Check sheet for the modelled part. Datum: model origin and axes. Units: mm. Face numbers are marked on the shaded views. Round coordinates to 2 decimals unless told otherwise and drop trailing zeros. Write each loop counter-clockwise with the first axis right and the second up, starting at its lowest first coordinate (ties: lowest second). Pieces come first, ordered by that corner, then holes. Notation, with made-up numbers: (16.25, 6) -> (44.25, 6) arc R20 ccw to (44.25, 44) -> close; hole circle Ø10 at (8, 52). An arc over 180 degrees is marked (long way). One line per item, written item: value.
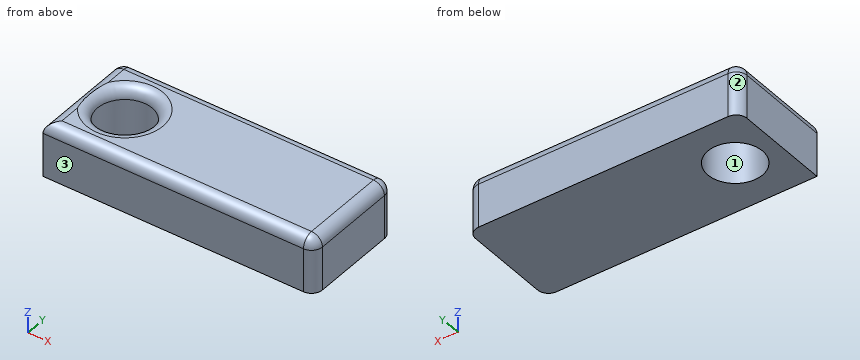
from build123d import *

# Parameters (mm, degrees)
F0_W         = 124.3421025574
F0_H         = 48.8486886024
F1_DEPTH     = 25
F3_D         = 25
F4_T1_DEPTH  = 149.3421025574
F4_T3_DEPTH  = 73.8486886024
F5_T1_DEPTH  = 32.5
F5_S5_W      = 5
F5_S5_H      = 5
F5_T6_DEPTH  = 5
F6_T1_DEPTH  = 32.5
F6_S5_W      = 5
F6_S5_H      = 5
F6_T6_DEPTH  = 5
F6_S11_W     = 5
F6_S11_H     = 5
F6_T12_DEPTH = 5


# Not quite as in the source:
# - a fillet or chamfer that OpenCascade refuses, or shapes differently, is made with other operations: its cross-section is extruded or revolved along the edge and cut away or added


with BuildPart() as f1:
    # F0 (on Top) → F1 (new body)
    with BuildSketch(Plane.XY):
        with Locations((-25.8323382586, 0)):
            Rectangle(F0_W, F0_H)
    extrude(amount=F1_DEPTH)

    # F3 (through all)
    with Locations(Plane.XY.offset(25)):
        with Locations((-68.3952495456, 0)):
            Hole(F3_D / 2)

    # F4: fillet of radius 5 on 5 edges, made by hand

    # F4_s2 → F4_t1 (cut)
    with BuildSketch(Plane.YZ.offset(-100.5033895373)):
        with BuildLine():
            ThreePointArc((24.4243443012, 20), (22.9598782072, 23.5355339059), (19.4243443012, 25))
            Line((19.4243443012, 25), (24.4243443012, 25))
            Line((24.4243443012, 25), (24.4243443012, 20))
        make_face()
        with BuildLine():
            ThreePointArc((-19.4243443012, 25), (-22.9598782072, 23.5355339059), (-24.4243443012, 20))
            Line((-24.4243443012, 20), (-24.4243443012, 25))
            Line((-24.4243443012, 25), (-19.4243443012, 25))
        make_face()
    extrude(amount=F4_T1_DEPTH, mode=Mode.SUBTRACT)

    # F4_s4 → F4_t3 (cut)
    with BuildSketch(Plane.XZ.offset(-36.9243443012)):
        with BuildLine():
            ThreePointArc((36.3387130201, 20), (34.874246926, 23.5355339059), (31.3387130201, 25))
            Line((31.3387130201, 25), (36.3387130201, 25))
            Line((36.3387130201, 25), (36.3387130201, 20))
        make_face()
        with BuildLine():
            ThreePointArc((-88.0033895373, 20), (-86.5389234433, 23.5355339059), (-83.0033895373, 25))
            Line((-83.0033895373, 25), (-88.0033895373, 25))
            Line((-88.0033895373, 25), (-88.0033895373, 20))
        make_face()
    extrude(amount=F4_T3_DEPTH, mode=Mode.SUBTRACT)

    # F4_s5 → F4_t6 (revolve, cut)
    with BuildSketch(Plane.XZ):
        with BuildLine():
            ThreePointArc((-50.8952495456, 25), (-54.4307834515, 23.5355339059), (-55.8952495456, 20))
            Line((-55.8952495456, 20), (-55.8952495456, 25))
            Line((-55.8952495456, 25), (-50.8952495456, 25))
        make_face()
    revolve(axis=Axis((-68.3952495456, 0, 25), (0, 0, 1)), mode=Mode.SUBTRACT)

    # F5: fillet of radius 5 on 1 edges, made by hand

    # F5_s2 → F5_t1 (cut)
    with BuildSketch(Plane.XY.offset(-12.5)):
        with BuildLine():
            ThreePointArc((36.3387130201, -19.4243443012), (34.874246926, -22.9598782072), (31.3387130201, -24.4243443012))
            Line((31.3387130201, -24.4243443012), (36.3387130201, -24.4243443012))
            Line((36.3387130201, -24.4243443012), (36.3387130201, -19.4243443012))
        make_face()
    extrude(amount=F5_T1_DEPTH, mode=Mode.SUBTRACT)


with BuildPart() as f5_tool4:
    # F5_s5 → F5_t6 (new body)
    with BuildSketch(Plane.YZ.offset(31.3387130201)):
        with Locations((-21.9243443012, 22.5)):
            Rectangle(F5_S5_W, F5_S5_H)
    extrude(amount=F5_T6_DEPTH)

    # F5_s7 → F5_t8 (revolve, cut)
    with BuildSketch(Plane(origin=(31.3387130201, -19.4243443012, 20), x_dir=(0, 0.7071067812, -0.7071067812), z_dir=(0, -0.7071067812, -0.7071067812))):
        with BuildLine():
            ThreePointArc((0, -5), (5, 0), (0, 5))
            Line((0, 5), (0, -5))
        make_face()
    revolve(axis=Axis((31.3387130201, -19.4243443012, 20), (1, 0, 0)), mode=Mode.SUBTRACT)


with BuildPart() as f1_1:
    add(f1.part)

    # F5_t3: cut F5_tool4
    add(f5_tool4.part, mode=Mode.SUBTRACT)

    # F6: fillet of radius 5 on 2 edges, made by hand

    # F6_s2 → F6_t1 (cut)
    with BuildSketch(Plane.XY.offset(-12.5)):
        with BuildLine():
            ThreePointArc((-83.0033895373, 24.4243443012), (-86.5389234433, 22.9598782072), (-88.0033895373, 19.4243443012))
            Line((-88.0033895373, 19.4243443012), (-88.0033895373, 24.4243443012))
            Line((-88.0033895373, 24.4243443012), (-83.0033895373, 24.4243443012))
        make_face()
        with BuildLine():
            ThreePointArc((31.3387130201, 24.4243443012), (34.874246926, 22.9598782072), (36.3387130201, 19.4243443012))
            Line((36.3387130201, 19.4243443012), (36.3387130201, 24.4243443012))
            Line((36.3387130201, 24.4243443012), (31.3387130201, 24.4243443012))
        make_face()
    extrude(amount=F6_T1_DEPTH, mode=Mode.SUBTRACT)


with BuildPart() as f6_tool4:
    # F6_s5 → F6_t6 (new body)
    with BuildSketch(Plane.XZ.offset(-19.4243443012)):
        with Locations((33.8387130201, 22.5)):
            Rectangle(F6_S5_W, F6_S5_H)
    extrude(amount=-F6_T6_DEPTH)

    # F6_s7 → F6_t8 (revolve, cut)
    with BuildSketch(Plane(origin=(31.3387130201, 19.4243443012, 20), x_dir=(-0.7071067812, 0, -0.7071067812), z_dir=(0.7071067812, 0, -0.7071067812))):
        with BuildLine():
            ThreePointArc((0, -5), (5, 0), (0, 5))
            Line((0, 5), (0, -5))
        make_face()
    revolve(axis=Axis((31.3387130201, 19.4243443012, 20), (0, 1, 0)), mode=Mode.SUBTRACT)


with BuildPart() as f1_2:
    add(f1_1.part)

    # F6_t3: cut F6_tool4
    add(f6_tool4.part, mode=Mode.SUBTRACT)


with BuildPart() as f6_tool10:
    # F6_s11 → F6_t12 (new body)
    with BuildSketch(Plane.XZ.offset(-19.4243443012)):
        with Locations((-85.5033895373, 22.5)):
            Rectangle(F6_S11_W, F6_S11_H)
    extrude(amount=-F6_T12_DEPTH)

    # F6_s13 → F6_t14 (revolve, cut)
    with BuildSketch(Plane(origin=(-83.0033895373, 19.4243443012, 20), x_dir=(0.7071067812, 0, -0.7071067812), z_dir=(0.7071067812, 0, 0.7071067812))):
        with BuildLine():
            ThreePointArc((0, -5), (5, 0), (0, 5))
            Line((0, 5), (0, -5))
        make_face()
    revolve(axis=Axis((-83.0033895373, 19.4243443012, 20), (0, 1, 0)), mode=Mode.SUBTRACT)


with BuildPart() as f1_3:
    add(f1_2.part)

    # F6_t9: cut F6_tool10
    add(f6_tool10.part, mode=Mode.SUBTRACT)


solid = f1_3.part
Item 1: Sectioned sample at A-A (z = 8). Enter the section's corners in (x, y), then the cut area to 3 significant figures.
Result set:
outline: (-88, -24.42) -> (31.34, -24.42) arc R5 ccw to (36.34, -19.42) -> (36.34, 19.42) arc R5 ccw to (31.34, 24.42) -> (-83, 24.42) arc R5 ccw to (-88, 19.42) -> close; hole circle Ø25 at (-68.4, 0)
area: 5,570 mm^2
Item 2: Sectioned sample at B-B (y = 0). Enter the section's corners in (x, z).
Result set:
outline: (-88, 0) -> (-80.9, 0) -> (-80.9, 20) arc R5 ccw to (-84.45, 24.79) arc R5 ccw to (-88, 20) -> close; (-55.9, 0) -> (36.34, 0) -> (36.34, 20) arc R5 ccw to (31.34, 25) -> (-50.9, 25) arc R5 ccw to (-55.9, 20) -> close
Item 3: Release check for a two-part mould opening along X. For the marked faces 1, 2 and 3 record: pulls with the +X half, pulls with the -X half, needs draft (parallel to the pull), parting line crosses it, or undercut.
Result set:
face 1: undercut
face 2: pulls with the -X half
face 3: needs draft
Item 4: Sectioned sample at C-C (z = 22.75). Enter the section's corners in (x, y).
Result set:
outline: (-87.18, -23.6) -> (31.34, -23.6) arc R4.18 ccw to (35.51, -19.42) -> (35.51, 19.42) arc R4.18 ccw to (31.34, 23.6) -> (-83, 23.6) arc R4.18 ccw to (-87.18, 19.42) -> close; hole circle Ø26.65 at (-68.4, 0)
Item 5: Material ranges on line 1 along X through (y, z) = (0, 10.25); line 2 along X through (y, z) = (-1.5, 12.5); line 3 along X through (y, z) = (-21.5, 17.5), recorded low to high.
Result set:
line 1: -88 to -80.9, -55.9 to 36.34
line 2: -88 to -80.8, -55.99 to 36.34
line 3: -88 to 35.89
